from build123d import *

# Parameters (mm, degrees)
SKETCH1_R           = 12.5
BOSS_EXTRUDE1_DEPTH = 40
BOSS_EXTRUDE2_DEPTH = 20
SKETCH3_W           = 30.675059353
SKETCH3_H           = 4.752473984
CUT_EXTRUDE1_DEPTH  = 15


with BuildPart() as part:
    # Sketch1 → Boss-Extrude1 (new body)
    with BuildSketch(Plane.XY):
        Circle(SKETCH1_R)
    extrude(amount=BOSS_EXTRUDE1_DEPTH)

    # Sketch2 → Boss-Extrude2 (add)
    with BuildSketch(Plane.XY.offset(40)):
        Polygon((20.501198272, 0), (10.250599136, 17.754558511), (-10.250599136, 17.754558511), (-20.501198272, 0), (-10.250599136, -17.754558511), (10.250599136, -17.754558511), align=None)
    extrude(amount=BOSS_EXTRUDE2_DEPTH)

    # Sketch3 → Cut-Extrude1 (cut)
    with BuildSketch(Plane.XY.offset(60)):
        with Locations((0.504050272, -0.180017954)):
            Rectangle(SKETCH3_W, SKETCH3_H)
    extrude(amount=-CUT_EXTRUDE1_DEPTH, mode=Mode.SUBTRACT)


solid = part.part
Could you check a few things on this model? Use its own coordinates, in mm. A direction names the side the tool comes from. Round coordinates to 2 decimals unless told otherwise and drop trailing zeros. Order: outer loops, then holes, each group sorted by start corner. A loop starts at its lowest first (then second) coordinate and runs counter-clockwise, first axis right, second up.
Q1. Imagine slicing it at A-A, the plane x = 0. List the corners of the cut face in (y, z) for me.
Geometry says:
outline: (-17.75, 40) - (-12.5, 40) - (-12.5, 0) - (12.5, 0) - (12.5, 40) - (17.75, 40) - (17.75, 60) - (2.2, 60) - (2.2, 45) - (-2.56, 45) - (-2.56, 60) - (-17.75, 60) - close
Q2. I'm going to push flat-ended pins straight in: P1, Ø1.4, axis at x = -3, y = 0.5, coming from the +Z side; P2, Ø4, axis at x = -7.5, z = 13, coming from the -Y side (3 decimals); P3, Ø5, axis at y = 0, z = 51, coming from the -X side; P4, Ø6, axis at x = -16.5, z = 12, coming from the +Y side. Where does each tip first touch, or does it pass through?
Geometry says:
P1: stops at z = 45
P2: stops at y = -11.225
P3: stops at x = -20.5
P4: passes through
Q3. Which directions (+Z, -Z, +X, -X, +Y, -Y) give clear straight access to the entire face, cutting with the end or side of a thin tool? Please do faces 1 (the face through (15.45, 8.75, 49.86)), 2 (the face through (11.923, 3.755, 19.72)), 3 (the face through (0, 0, 45)).
Geometry says:
face 1: +Z, -Z, +X, +Y
face 2: -Z
face 3: +Z
Q4. Imagine slicing it at B-B, the plane y = -6. List the corners of the cut face in (x, z) for me.
Geometry says:
outline: (-17.04, 40) - (-10.97, 40) - (-10.97, 0) - (10.97, 0) - (10.97, 40) - (17.04, 40) - (17.04, 60) - (-17.04, 60) - close
Q5. Imagine slicing it at C-C, the plane z = 29. List the corners of the cut face in (x, y) for me, then the cut area to 3 significant figures.
Geometry says:
outline: circle Ø25 at (0, 0)
area: 491 mm2
Q6. Thinking about a two-plate mould opening in Y: for faces 4 (the face through (-15.304, 9.002, 49.86)), 5 (the face through (0, -2.556, 53)), 6 (the face through (0, 4, 60)), which applies, released by +Y, released by -Y, zero draft, split by the parting line, or undercut?
Geometry says:
face 4: released by +Y
face 5: undercut
face 6: zero draft
Q7. Please list where these lines run through material, in increasing order: probe 1 along Z at (x, y) = (5.5, 1.5); probe 2 along Y at (x, z) = (-8.5, 49.5); probe 3 along X at (y, z) = (-2.5, 48.5).
Geometry says:
probe 1: z = 0 to 45
probe 2: y = -17.75 to -2.56, 2.2 to 17.75
probe 3: x = -19.06 to -14.83, 15.84 to 19.06
Q8. Imagine slicing it at D-D, the plane x = 5. List the corners of the cut face in (y, z) for me, then the cut area to 3 significant figures.
Geometry says:
outline: (-17.75, 40) - (-11.46, 40) - (-11.46, 0) - (11.46, 0) - (11.46, 40) - (17.75, 40) - (17.75, 60) - (2.2, 60) - (2.2, 45) - (-2.56, 45) - (-2.56, 60) - (-17.75, 60) - close
area: 1,560 mm2
